Geometry check sheet. Reference: drawing and pictorial views, mm from the part's lowest x, y, z. Round coordinates to 2 decimals unless told otherwise and drop trailing zeros. Order: outer loops, then holes, each group sorted by start corner. A loop starts at its lowest first (then second) coordinate and runs counter-clockwise, first axis right, second up. Notation, with made-up numbers: (52, 55) -> (60, 55) arc R34 ccw to (60, 86) -> close; hole circle Ø3 at (51.25, 28). An arc over 180 degrees is marked (long way). Return JSON: item names as keys, results as strings. Group by question number.
1) Scan lines: L1, parallel to X at y = 5.25, z = 19.5 (1 decimal); L2, parallel to Y at x = 3.25, z = 48 (1 decimal); L3, parallel to X at y = 2.5, z = 19. Record each from-to range of solid material in increasing order.
2) Section check C-C on x = 15.25. Enter the section's corners in (y, z) (1 decimal).
3) Depth check by flat-ended pin: pin 1 (2 mm diameter, centred on x = 3, y = 2.5, fed in from +Z) (1 decimal); pin 2 (0.5 mm diameter, centred on y = 3.5, z = 34.5, fed in from -X); pin 3 (1.5 mm diameter, centred on x = 15.5, z = 31, fed in from +Y). Enter the tip coordinate at first touch or a pass-through.
4) Section check B-B on z = 40.5. Enter the section's corners in (x, y) (1 decimal), plus the area to 3 significant figures.
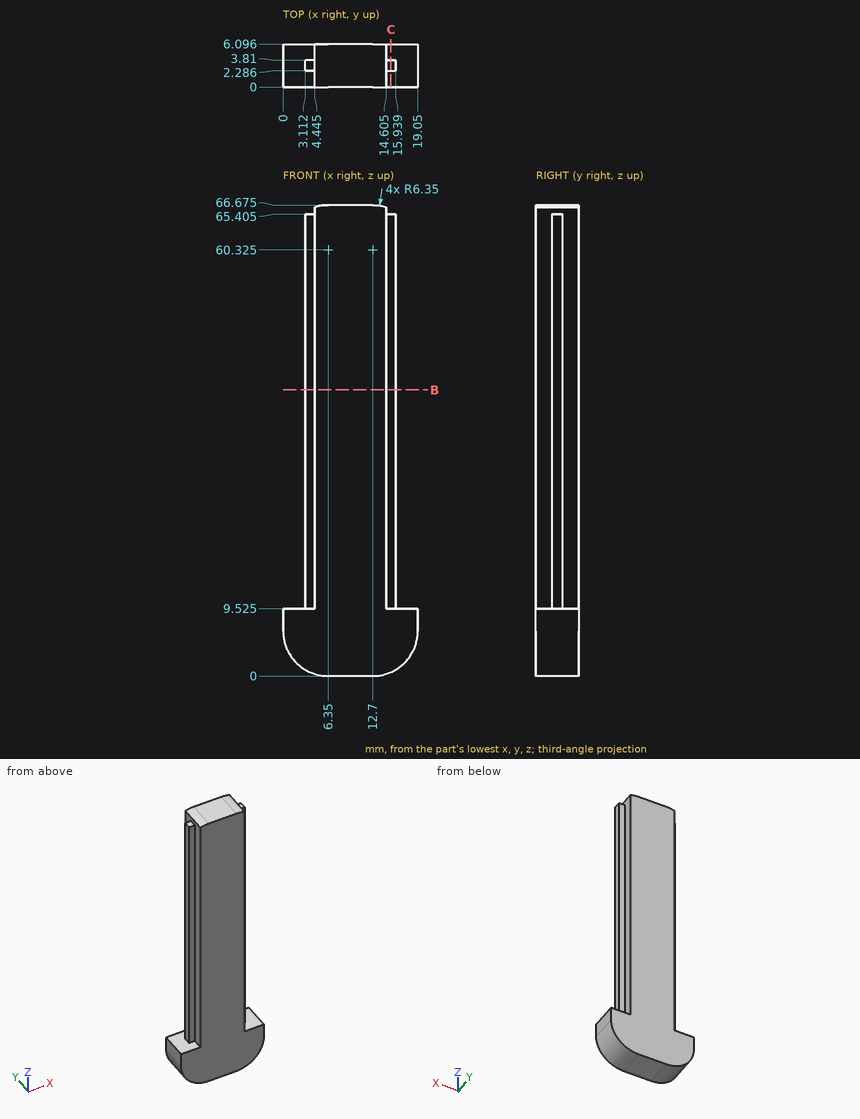
Check result:
{
 "1": {"L1": "4.4 to 14.6", "L2": "2.3 to 3.8", "L3": "3.11 to 15.94"},
 "2": {"outline": "(0, 0.5) -> (6.1, 0.5) -> (6.1, 9.5) -> (3.8, 9.5) -> (3.8, 65.4) -> (2.3, 65.4) -> (2.3, 9.5) -> (0, 9.5) -> close"},
 "3": {"pin 1": "z = 65.4", "pin 2": "x = 3.11", "pin 3": "y = 3.81"},
 "4": {"outline": "(3.1, 2.3) -> (4.4, 2.3) -> (4.4, 0) -> (14.6, 0) -> (14.6, 2.3) -> (15.9, 2.3) -> (15.9, 3.8) -> (14.6, 3.8) -> (14.6, 6.1) -> (4.4, 6.1) -> (4.4, 3.8) -> (3.1, 3.8) -> close", "area": "66.0 mm^2"}
}
